```python
from build123d import *

# Parameters (mm, degrees)
SKETCH1_W              = 30
SKETCH1_H              = 35.1
BOSS_EXTRUDE1_DEPTH    = 6
CHAMFER1_SIZE          = 10
M5_CLEARANCE_HOLE1_D   = 5.3
SKETCH234_W            = 10
SKETCH234_H            = 6
BOSS_EXTRUDE234_DEPTH  = 6
FILLET134_R            = 1
SKETCH2341_W           = 10
SKETCH2341_H           = 6
BOSS_EXTRUDE2341_DEPTH = 6
FILLET1341_R           = 1
FILLET1342_R           = 10


with BuildPart() as part:
    # Sketch1 → Boss-Extrude1 (new body)
    with BuildSketch(Plane(origin=(0, 0, 0), x_dir=(1, 0, 0), z_dir=(0, 1, 0))):
        with Locations((15, 17.55)):
            Rectangle(SKETCH1_W, SKETCH1_H)
    extrude(amount=BOSS_EXTRUDE1_DEPTH)

    # Chamfer1
    chamfer1_edges = [part.edges().sort_by_distance(p)[0] for p in [
        (30, 3, -35.1),
        (30, 3, 0),
    ]]
    chamfer(chamfer1_edges, length=CHAMFER1_SIZE)

    # M5 Clearance Hole1 (through all)
    with Locations(Plane(origin=(0, 0, 0), x_dir=(-1, 0, 0), z_dir=(0, -1, 0))):
        with Locations((-15, 14)):
            Hole(M5_CLEARANCE_HOLE1_D / 2)

    # Sketch234 → Boss-Extrude234 (add)
    with BuildSketch(Plane(origin=(0, 6, -8.007221392), x_dir=(0, 0, -1), z_dir=(-1, 0, 0))):
        with Locations((0.767778608, 3)):
            Rectangle(SKETCH234_W, SKETCH234_H)
    extrude(amount=BOSS_EXTRUDE234_DEPTH)

    # Fillet134
    fillet134_edges = [part.edges().sort_by_distance(p)[0] for p in [
        (-6, 3, -3.775),
        (-6, 3, -13.775),
    ]]
    fillet(fillet134_edges, radius=FILLET134_R)

    # Sketch2341 → Boss-Extrude2341 (add)
    with BuildSketch(Plane(origin=(0, 0, -27.092778608), x_dir=(0, 0, 1), z_dir=(-1, 0, 0))):
        with Locations((0.767778608, 3)):
            Rectangle(SKETCH2341_W, SKETCH2341_H)
    extrude(amount=BOSS_EXTRUDE2341_DEPTH)

    # Fillet1341
    fillet1341_edges = [part.edges().sort_by_distance(p)[0] for p in [
        (-6, 3, -21.325),
        (-6, 3, -31.325),
    ]]
    fillet(fillet1341_edges, radius=FILLET1341_R)

    # Fillet1342
    fillet1342_edges = [part.edges().sort_by_distance(p)[0] for p in [
        (20, 3, -35.1),
        (30, 3, -10),
        (30, 3, -25.1),
        (20, 3, 0),
    ]]
    fillet(fillet1342_edges, radius=FILLET1342_R)


solid = part.part
```
Design review of the part built by this model. Coordinates are the model's own, in mm. A direction names the side the tool comes from. Coordinates: 2 decimals unless noted, no trailing zeros. Order: outer loops, then holes, each group sorted by start corner. A loop starts at its lowest first (then second) coordinate and runs counter-clockwise, first axis right, second up. Notation, with made-up numbers: (0, -3.5) -> (8, -3.5) arc R20 cw to (8, 10.5) -> close; hole circle Ø7 at (-14.75, -12). An arc over 180 degrees is marked (long way). One line per item, written item: value. Start each with the question number.
Q1. Take a section at A-A, the plane x = 15. State the section outline as (y, z) points.
Q2. Tool access review of faces 1 (the flat face through (-2, 3, -3.775)), 2 (the cylindrical face through (-5.7, 3.04, -31.04)), 3 (the flat face through (0, 3, -17)): name each direction out of +Z, -Z, +X, -X, +Y, -Y from which nothing blocks a thin tool from reaching the whole face with its end or side.
Q3. Take a section at B-B, the plane y = 2. State the section outline as (x, z) points (3 decimals).
Q4. Take a section at D-D, the plane z = -20.5. State the section outline as (x, y) points.
Q5. Insertion check: pin 1 Ø6 at (x, z) = (17.5, -11) entering from -Y; pin 2 Ø1.5 at (x, y) = (-2, 3) entering from -Z (3 decimals); pin 3 Ø3 at (x, y) = (26, 5) entering from +Z; pin 4 Ø3 at (y, z) = (1.5, -2.5) entering from -X. Each pin has a flat end and moves straight along its axis. Give the tip position at first contact, or say it passes through.
Q6. For probe 1 along X at (y, z) = (1.35, -14); probe 2 along Z at (x, y) = (15, 1.8); probe 3 along X at (y, z) = (3.4, -19.5), list the stretches that pass through material, from the lowest coordinate up.
Q7. Take a section at C-C, the plane x = -1. State the section outline as (y, z) points (3 decimals), then the cut area to 3 significant figures.
Values follow:
1. outline: (0, -35.1) -> (6, -35.1) -> (6, -16.65) -> (0, -16.65) -> close; (0, -11.35) -> (6, -11.35) -> (6, 0) -> (0, 0) -> close
2. face 1: +Z, -X, +Y, -Y
2. face 2: -Z, -X, +Y, -Y
2. face 3: -X, +Y, -Y
3. outline: (-6, -30.325) arc R1 ccw to (-5, -31.325) -> (0, -31.325) -> (0, -35.1) -> (15.858, -35.1) arc R10 ccw to (22.929, -32.171) -> (27.071, -28.029) arc R10 ccw to (30, -20.958) -> (30, -14.142) arc R10 ccw to (27.071, -7.071) -> (22.929, -2.929) arc R10 ccw to (15.858, 0) -> (0, 0) -> (0, -3.775) -> (-5, -3.775) arc R1 ccw to (-6, -4.775) -> (-6, -12.775) arc R1 ccw to (-5, -13.775) -> (0, -13.775) -> (0, -21.325) -> (-5, -21.325) arc R1 ccw to (-6, -22.325) -> close; hole circle Ø5.3 at (15, -14)
4. outline: (0, 0) -> (30, 0) -> (30, 6) -> (0, 6) -> close
5. pin 1: stops at y = 0
5. pin 2: stops at z = -31.325
5. pin 3: stops at z = -4.5
5. pin 4: stops at x = -5.63
6. probe 1: x = 0 to 12.35, 17.65 to 30
6. probe 2: z = -35.1 to -16.65, -11.35 to 0
6. probe 3: x = 0 to 30
7. outline: (0, -31.325) -> (6, -31.325) -> (6, -21.325) -> (0, -21.325) -> close; (0, -13.775) -> (6, -13.775) -> (6, -3.775) -> (0, -3.775) -> close
7. area: 120 mm2
